Build history of the part. All positions in model axes, mm. Give positions to 0.01 mm unless a question says otherwise; leave off trailing zeros. Answer in a Markdown table with one row per item. Add a question column.
from build123d import *

# Parameters (mm, degrees)
F0_R     = 2.5
F2_DEPTH = 412


with BuildPart() as f2:
    # F0 (on Front) → F2 (new body)
    with BuildSketch(Plane.XZ):
        with BuildLine():
            Line((6.5, 0), (2, 0))
            ThreePointArc((2, 0), (0.5857864376, -0.5857864376), (0, -2))
            Line((0, -2), (0, -6.4857100192))
            Line((0, -6.4857100192), (0.4948230833, -6.489995392))
            Line((0.4948230833, -6.489995392), (0.4948230833, -7))
            Line((0.4948230833, -7), (2, -7))
            Line((2, -7), (2, -3.0833937817))
            Line((2, -3.0833937817), (6.2, -7.2637052917))
            Line((6.2, -7.2637052917), (6.2, -12.7393398282))
            Line((6.2, -12.7393398282), (2, -16.9393398282))
            Line((2, -16.9393398282), (2, -13))
            Line((2, -13), (0.5, -13))
            Line((0.5, -13), (0.5, -13.5))
            Line((0.5, -13.5), (0, -13.5))
            Line((0, -13.5), (0, -26.4857100192))
            Line((0, -26.4857100192), (0.4948230833, -26.489995392))
            Line((0.4948230833, -26.489995392), (0.4948230833, -27))
            Line((0.4948230833, -27), (2, -27))
            Line((2, -27), (2, -23.0833937817))
            Line((2, -23.0833937817), (6.2, -27.2637052917))
            Line((6.2, -27.2637052917), (6.2, -32.7393398282))
            Line((6.2, -32.7393398282), (2, -36.9393398282))
            Line((2, -36.9393398282), (2, -33))
            Line((2, -33), (0.5, -33))
            Line((0.5, -33), (0.5, -33.5))
            Line((0.5, -33.5), (0, -33.5))
            Line((0, -33.5), (0, -38))
            ThreePointArc((0, -38), (0.5857864376, -39.4142135624), (2, -40))
            Line((2, -40), (6.5, -40))
            Line((6.5, -40), (6.5, -39.5))
            Line((6.5, -39.5), (7, -39.5))
            Line((7, -39.5), (7, -38))
            Line((7, -38), (3.0606601718, -38))
            Line((3.0606601718, -38), (7.2606601718, -33.8))
            Line((7.2606601718, -33.8), (12.7393398282, -33.8))
            Line((12.7393398282, -33.8), (16.9393398282, -38))
            Line((16.9393398282, -38), (13.015800612, -38))
            Line((13.015800612, -38), (13.015800612, -39.5))
            Line((13.015800612, -39.5), (13.5, -39.5))
            Line((13.5, -39.5), (13.5, -40))
            Line((13.5, -40), (18, -40))
            ThreePointArc((18, -40), (19.4142135624, -39.4142135624), (20, -38))
            Line((20, -38), (20, -33.4626608249))
            Line((20, -33.4626608249), (19.5363645284, -33.4624647606))
            Line((19.5363645284, -33.4624647606), (19.532302618, -32.9822008219))
            Line((19.532302618, -32.9822008219), (18, -32.9822008219))
            Line((18, -32.9822008219), (17.9998106987, -36.9393398192))
            Line((17.9998106987, -36.9393398192), (13.8264202785, -32.765949399))
            Line((13.8264202785, -32.765949399), (13.8264202785, -27.246708479))
            Line((13.8264202785, -27.246708479), (17.9998106987, -23.0606601627))
            Line((17.9998106987, -23.0606601627), (17.9998106987, -26.9999999909))
            Line((17.9998106987, -26.9999999909), (19.4998106987, -26.9999999909))
            Line((19.4998106987, -26.9999999909), (19.4998106987, -26.4999999909))
            Line((19.4998106987, -26.4999999909), (20, -26.4999999909))
            Line((20, -26.4999999909), (20, -13.4626608249))
            Line((20, -13.4626608249), (19.5363645284, -13.4624647606))
            Line((19.5363645284, -13.4624647606), (19.532302618, -12.9822008219))
            Line((19.532302618, -12.9822008219), (18, -12.9822008219))
            Line((18, -12.9822008219), (17.9998106987, -16.9393398192))
            Line((17.9998106987, -16.9393398192), (13.8264202785, -12.765949399))
            Line((13.8264202785, -12.765949399), (13.8264202785, -7.246708479))
            Line((13.8264202785, -7.246708479), (17.9998106987, -3.0606601627))
            Line((17.9998106987, -3.0606601627), (17.9998106987, -6.9999999909))
            Line((17.9998106987, -6.9999999909), (19.4998106987, -6.9999999909))
            Line((19.4998106987, -6.9999999909), (19.4998106987, -6.4999999909))
            Line((19.4998106987, -6.4999999909), (20, -6.4999999909))
            Line((20, -6.4999999909), (20, -2))
            ThreePointArc((20, -2), (19.4142135624, -0.5857864376), (18, 0))
            Line((18, 0), (13.4962801728, 0.0202495232))
            Line((13.4962801728, 0.0202495232), (13.5, -0.5))
            Line((13.5, -0.5), (13.015800612, -0.5))
            Line((13.015800612, -0.5), (13.015800612, -2))
            Line((13.015800612, -2), (16.9393398282, -2))
            Line((16.9393398282, -2), (12.7393121854, -6.2000276428))
            Line((12.7393121854, -6.2000276428), (7.2606601718, -6.2))
            Line((7.2606601718, -6.2), (3.0606601718, -2))
            Line((3.0606601718, -2), (7, -2))
            Line((7, -2), (7, -0.5))
            Line((7, -0.5), (6.5, -0.5))
            Line((6.5, -0.5), (6.5, 0))
        make_face()
        with Locations((10, -30)):
            Circle(F0_R, mode=Mode.SUBTRACT)
        Polygon((7.2606601718, -13.8), (12.7393398282, -13.8), (16.9393398282, -18), (16.9393398282, -22), (12.7393121854, -26.2000276428), (7.2606601718, -26.2), (3.0606601718, -22), (3.0606601718, -18), align=None, mode=Mode.SUBTRACT)
        with Locations((10, -10)):
            Circle(F0_R, mode=Mode.SUBTRACT)
    extrude(amount=F2_DEPTH)


solid = f2.part
(1) Wall check: line 1 along Z through (x, y) = (10, -298); line 2 along Z through (x, y) = (18.25, -220.5); line 3 along X through (y, z) = (-183, -1.5). Give the ranges that are in metal, low to high. Write a range as from..to.
(2) Saw through at A-A, the plane y = -308. State how many separate pieces and enclosed holes the cut face has, then the cut area to 3 significant figures.
(3) Flat gauge pins, fed straight in: pin 1 Ø0.6 at (y, z) = (-215, -13) entering from -X; pin 2 Ø2 at (y, z) = (-155.5, -31) entering from -X; pin 3 Ø1.7 at (x, y) = (19, -185) entering from +Z. Where does each tip first touch, or does it go through?
Worked answers:
| question | item | result |
|---|---|---|
| 1 | line 1 | -33.8..-32.5, -27.5..-26.2, -13.8..-12.5, -7.5..-6.2 |
| 1 | line 2 | -39.98..-32.98, -27..-12.98, -7..-0.02 |
| 1 | line 3 | 0.06..7, 13.02..19.94 |
| 2 | separate pieces | 1 |
| 2 | enclosed holes | 3 |
| 2 | area | 302 mm^2 |
| 3 | pin 1 | x = 0.5 |
| 3 | pin 2 | x = 6.2 |
| 3 | pin 3 | z = -0.01 |
